Can you work these out from the drawing? Everything is in mm from the part's minimum corner. A direction names the side the tool comes from. Coordinates: 2 decimals unless noted, no trailing zeros. Order: outer loops, then holes, each group sorted by start corner. A loop starts at its lowest first (then second) coordinate and runs counter-clockwise, first axis right, second up. Notation, with made-up numbers: (23, 75.5) - (34, 75.5) arc R14 cw to (34, 99.5) - close; hole circle Ø1 at (33.5, -26.5). An arc over 180 degrees is marked (long way). One line per item, written item: value.
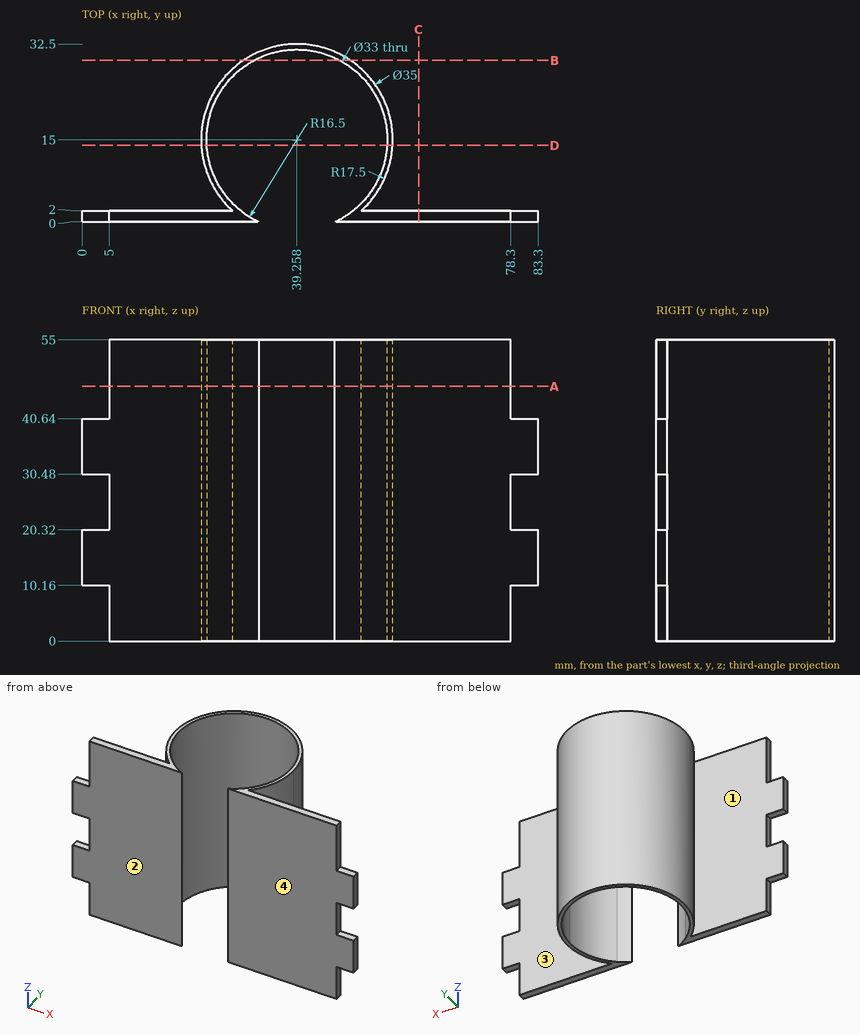
Item 1: I want a section at A-A on z = 46.5. Please give me the cut outline in (x, y).
Conclusion:
outline: (5, 0) - (32.38, 0) arc R16.5 cw (long way) to (46.13, 0) - (78.3, 0) - (78.3, 2) - (50.97, 2) arc R17.5 ccw (long way) to (27.54, 2) - (5, 2) - close
Item 2: I want a section at D-D on y = 14. Please give me the cut outline in (x, z), then the cut area to 3 significant figures.
Conclusion:
outline: (21.79, 0) - (22.79, 0) - (22.79, 55) - (21.79, 55) - close; (55.73, 0) - (56.73, 0) - (56.73, 55) - (55.73, 55) - close
area: 110 mm²
Item 3: I'm going to push flat-ended pins straight in: pin 1 Ø8 at (x, z) = (46.5, 35) entering from +Y; pin 2 Ø1 at (x, y) = (81, 1) entering from -Z; pin 3 Ø2 at (y, z) = (1.5, 48.5) entering from +X. Where does each tip first touch, or does it pass through?
Conclusion:
pin 1: y = 32.2
pin 2: z = 10.16
pin 3: x = 78.3
Item 4: For the marked faces 1 and 2, which set-ups out of +Z, -Z, +X, -X, +Y, -Y let a thin tool reach every point of the face, with its end or its side?
Conclusion:
face 1: +Z, -Z, -X
face 2: +Z, -Z, +X, -X, -Y
Item 5: I want a section at C-C on x = 61.5. Please give me the cut outline in (y, z).
Conclusion:
outline: (0, 0) - (2, 0) - (2, 55) - (0, 55) - close
Item 6: If I drill on probe 1 along X at (y, z) = (28, 22.5) (1 decimal); probe 2 along Y at (x, z) = (18, 47); probe 3 along X at (y, z) = (4, 3.5) (1 decimal), over which ranges is the centre line in solid material (lowest first)?
Conclusion:
probe 1: 27.5 to 29.1, 49.4 to 51
probe 2: 0 to 2
probe 3: 25.6 to 27, 51.6 to 52.9
Item 7: Thinking about a two-plate mould opening in Y: for the marked faces 3 and 4, which applies, pulls with the +Y half, pulls with the -Y half, needs draft (parallel to the pull), parting line crosses it, or undercut?
Conclusion:
face 3: undercut
face 4: pulls with the -Y half
Item 8: I want a section at B-B on y = 29.5. Please give me the cut outline in (x, z) (1 decimal).
Conclusion:
outline: (29.5, 0) - (31.4, 0) - (31.4, 55) - (29.5, 55) - close; (47.1, 0) - (49.1, 0) - (49.1, 55) - (47.1, 55) - close
